Input: part model. Units: mm. Frame: model coordinates. A direction names the side the tool comes from. Coordinates: 2 decimals unless noted, no trailing zeros. Loops run counter-clockwise (first coordinate to the right, second up) from the corner with the lowest first, then second, coordinate; pieces in that order, holes last. Notation, with made-up numbers: (61, 42.5) - (68, 42.5) arc R9 cw to (68, 46.5) - close; hole circle Ø4 at (75.25, 61). An arc over 180 degrees is marked (long way). Use a Markdown table: item, result. Add a question column.
1. Draft query along X for faces 1 (the face through (-27.6, 1.5, 6.8)), 2 (the face through (57.422, 8.065, 4.662)), 3 (the face through (-1, 8, 0)). Return one class per face: released by +X, released by -X, zero draft, split by the parting line, or undercut.
2. Section query C-C on x = 14. Return the cut outline in (y, z), then the cut area to 3 significant figures.
3. Contact query for flat-ended pins moving along their axis: P1, Ø6, axis at x = -40, y = 1.5, coming from the +Z side; P2, Ø4, axis at x = 25.5, y = 7, coming from the -Z side; P3, Ø3, axis at x = 37, z = 3.5, coming from the -Y side; P4, Ø5, axis at x = 18.5, y = 8, coming from the +Z side. Output: stop coordinate, or through.
4. Ray query, L1, parallel to X at y = 8.25, z = 5; L2, parallel to Z at x = 60, y = 8.2; L3, parallel to Z at x = -16, y = 7. Return the intervals inside material, ascending. Write a range as [from, to].
5. Access query for faces 4 (the face through (22.5, 4, 5)), 5 (the face through (-1, 8, 10)), 6 (the face through (-22.5, 4, 5)), 7 (the face through (64, 8, 2)). Directions: +Z, -Z, +X, -X, +Y, -Y. A direction counts if a zero-diameter tool reaches every point of the face in a straight line with its end or side. Return the directions, or none.
6. Section query B-B on y = 7. State how many separate pieces and enclosed holes the cut face has, then the cut area to 3 significant figures.
7. Section query A-A on x = -28. Return the cut outline in (y, z).
8. Section query D-D on z = -38. Return the cut outline in (x, y).
Autodesk Inventor part; units mm, degrees
ref_plane "YZ Plane" through (0, 0, 0) normal (1, 0, 0) x (0, 1, 0)
ref_plane "XZ Plane" through (0, 0, 0) normal (0, 1, 0) x (-1, 0, 0)
ref_plane "XY Plane" through (0, 0, 0) normal (0, 0, 1) x (1, 0, 0)
sketch "Sketch1" plane through (0, 0, 0) normal (0, 1, 0) x (-1, 0, 0)
  line L0 (0, -66) -> (0, 81)
  line L1 (-49, 0) -> (49, 0)
  line L2 (-35, -45) -> (35, -45)
  line L3 (20, 60) -> (-20, 60)
  line L4 (-20, 60) -> (-35, -45)
  line L5 (35, -45) -> (20, 60)
  point P0 (0, 0)
  dimension "d0" = 70
  dimension "d1" = 105
  dimension "d3" = 40
  dimension "d6" = 45
extrude "Extrusion1" add sketch "Sketch1" along normal blind 3
sketch "Sketch2" plane through (0, 0, 0) normal (0, 0, 1) x (1, 0, 0)
  line L0 (-91, 0) -> (91, 0)
  line L1 (0, 12.72) -> (0, -2.12)
  line L2 (35, 3) -> (-35, 3)
  line L3 (22.5, 3) -> (-22.5, 3)
  line L4 (-22.5, 3) -> (-22.5, 5.6)
  line L5 (22.5, 5.6) -> (22.5, 3)
  line L6 (22.5, 5.6) -> (65, 5.6)
  line L7 (65, 5.6) -> (65, 10.6)
  line L8 (65, 10.6) -> (-65, 10.6)
  line L9 (-65, 10.6) -> (-65, 5.6)
  line L10 (-65, 5.6) -> (-22.5, 5.6)
  line L11 (-35, 0) -> (-35, 3)
  line L12 (35, 0) -> (35, 3)
  point P0 (0, 0)
  point P1 (-22.5, 3)
  point P2 (22.5, 3)
  dimension "d8" = 2.6
  dimension "d9" = 130
  dimension "d10" = 5
  dimension "d11" = 2.6
  dimension "d22" = 45
extrude "Extrusion2" add sketch "Sketch2" along normal blind 10 contours L2 L4 L10 L9 L8 L1 | L1 L8 L7 L6 L5 L2
fillet "Fillet1" radius 5 4 edges at (65, 8.1, 0) (65, 8.1, 10) (-65, 8.1, 0) (-65, 8.1, 10)
sketch "Sketch3" plane through (-60, 10.6, 0) normal (0, 1, 0) x (1, 0, 0)
  arc A0 (0, 0) -> (0, -10) centre (0, -5) ccw
  arc A1 (120, -10) -> (120, 0) centre (120, -5) ccw
  point P0 (60, 0)
hole "Hole1" at (60, 10.6, 5) at (-60, 10.6, 5) direction (0, -1, 0) diameter 5.2 end through all
properties part number "karoserie2"
Resolved:
| question | item | result |
|---|---|---|
| 1 | face 1 | released by -X |
| 1 | face 2 | undercut |
| 1 | face 3 | zero draft |
| 2 | outline | (0, -45) - (3, -45) - (3, 0) - (10.6, 0) - (10.6, 10) - (3, 10) - (3, 60) - (0, 60) - close |
| 2 | area | 391 mm² |
| 3 | P1 | through |
| 3 | P2 | z = 0 |
| 3 | P3 | y = 5.6 |
| 3 | P4 | z = 10 |
| 4 | L1 | [-65, -62.6], [-57.4, 57.4], [62.6, 65] |
| 4 | L2 | [0, 2.4], [7.6, 10] |
| 4 | L3 | [0, 10] |
| 5 | face 4 | +Z, -Z, +X |
| 5 | face 5 | +Z, +X, -X, +Y |
| 5 | face 6 | +Z, -Z, -X |
| 5 | face 7 | -Z, +X, +Y, -Y |
| 6 | separate pieces | 1 |
| 6 | enclosed holes | 2 |
| 6 | area | 1,240 mm² |
| 7 | outline | (0, -45) - (3, -45) - (3, 4) - (0, 4) - close; (5.6, 0) - (10.6, 0) - (10.6, 10) - (5.6, 10) - close |
| 8 | outline | (-34, 0) - (34, 0) - (34, 3) - (-34, 3) - close |
